Check sheet for the modelled part. Datum: model origin and axes. Units: mm. A direction names the side the tool comes from. Coordinates: 2 decimals unless noted, no trailing zeros. Order: outer loops, then holes, each group sorted by start corner. A loop starts at its lowest first (then second) coordinate and runs counter-clockwise, first axis right, second up. Notation, with made-up numbers: M 11,46 L 16,46 A29 cw 16,79 Z; hole C -1,-4 d1. An arc over 180 degrees is marked long. Answer in a Markdown table with one row per item. Add a question column.
from build123d import *

# Parameters (mm, degrees)
BOSS_EXTRUDE1_DEPTH = 5
FILLET1_SIZE        = 20
FILLET1_SIZE_2      = 5
FILLET2_R           = 2
FILLET3_R           = 5


with BuildPart() as part:
    # Sketch1 → Boss-Extrude1 (new body)
    with BuildSketch(Plane(origin=(0, 0, 0), x_dir=(1, 0, 0), z_dir=(0, 1, 0))):
        Polygon((0, 0), (55, 0), (55, -38.6), (0, -38.6), (0, -34.6), (-3, -34.6), (-3, -41.6), (1.5, -41.6), (58, -41.6), (58, 3), (0, 3), (-3, 3), (-3, -4), (0, -4), align=None)
    extrude(amount=BOSS_EXTRUDE1_DEPTH)

    # Fillet1
    # an asymmetric fillet: 20, 5 mm, written as the material it adds along each edge
    with BuildSketch(Plane(origin=(55, 0, 0), x_dir=(-1, 0, 0), z_dir=(0, 1, 0))) as fillet1_piece_1:
        with BuildLine():
            Bezier((FILLET1_SIZE, 0), (0, 0), (0, FILLET1_SIZE_2), weights=[1, 0.707106781, 1])
            Line((0, FILLET1_SIZE_2), (0, 0))
            Line((0, 0), (FILLET1_SIZE, 0))
        make_face()
    extrude(amount=5)
    with BuildSketch(Plane(origin=(55, 0, 38.6), x_dir=(-1, 0, 0), z_dir=(0, 1, 0))) as fillet1_piece_2:
        with BuildLine():
            Bezier((FILLET1_SIZE, 0), (0, 0), (0, -FILLET1_SIZE_2), weights=[1, 0.707106781, 1])
            Line((0, -FILLET1_SIZE_2), (0, 0))
            Line((0, 0), (FILLET1_SIZE, 0))
        make_face()
    extrude(amount=5)

    # Fillet2
    fillet2_edges = [part.edges().sort_by_distance(p)[0] for p in [
        (-3, 2.5, 4),
        (-3, 2.5, -3),
        (-3, 2.5, 41.6),
        (-3, 2.5, 34.6),
    ]]
    fillet(fillet2_edges, radius=FILLET2_R)

    # Fillet3
    fillet3_edges = [part.edges().sort_by_distance(p)[0] for p in [
        (58, 2.5, -3),
        (58, 2.5, 41.6),
    ]]
    fillet(fillet3_edges, radius=FILLET3_R)


solid = part.part
1. Set-up check for faces 5 (the flat face through (55, 2, 19)), 6 (the flat face through (18, 2, 38.6)), 7 (the flat face through (26, 2, 41.6)): record each of +Z, -Z, +X, -X, +Y, -Y from which the full face is reachable in a straight line by a thin tool's end or side.
2. Section check B-B on z = 23.5. Enter the section's corners in (x, y), then the cut area to 3 significant figures.
3. Go/stop test with flat-tipped pins: pin 1 Ø1.5 at (y, z) = (2, 15) entering from -X; pin 2 Ø12 at (x, z) = (36, 9.5) entering from +Y. Record where each tip stops, or that it passes through.
4. Scan lines: line 1 (Z direction, x = 26.5, y = 0.55); line 2 (X direction, y = 1.4, z = 8); line 3 (Z direction, x = 39, y = 2.6). Record each from-to range of solid material in increasing order.
5. Release check for a two-part mould opening along Z. For faces 1 (the flat face through (58, 2, 20)), 2 (the flat face through (0, 2, 2)), 3 (the flat face through (0, 2, 37)), 4 (the cylindrical face through (56, 3, -2)) record: released by +Z, released by -Z, zero draft, split by the parting line, or undercut.
6. Section check A-A on x = 30.5. Enter the section's corners in (y, z), then the cut area to 3 significant figures.
Result sheet:
| question | item | result |
|---|---|---|
| 1 | face 5 | -X, +Y, -Y |
| 1 | face 6 | +Y, -Y |
| 1 | face 7 | +Z, +X, -X, +Y, -Y |
| 2 | outline | M 55,0 L 58,0 L 58,5 L 55,5 Z |
| 2 | area | 15.0 mm^2 |
| 3 | pin 1 | x = 55 |
| 3 | pin 2 | through |
| 4 | line 1 | -3 to 0, 38.6 to 41.6 |
| 4 | line 2 | 55 to 58 |
| 4 | line 3 | -3 to 0.1, 38.5 to 41.6 |
| 5 | face 1 | zero draft |
| 5 | face 2 | undercut |
| 5 | face 3 | undercut |
| 5 | face 4 | released by -Z |
| 6 | outline | M 0,-3 L 5,-3 L 5,0 L 0,0 Z; M 0,38.6 L 5,38.6 L 5,41.6 L 0,41.6 Z |
| 6 | area | 30.0 mm^2 |
